```python
from build123d import *

# Parameters (mm, degrees)
CYLINDER028_R           = 1.1
CYLINDER028_DEPTH       = 10
CYLINDER031_R           = 0.9
CYLINDER031_DEPTH       = 10
CYLINDER029_R           = 2.5
CYLINDER029_DEPTH       = 3.5
CYLINDER030_R           = 2
CYLINDER030_DEPTH       = 5.2
LINK011_PLACEMENT_ANGLE = 90
LINK012_PLACEMENT_ANGLE = 90
CYLINDER027_R           = 1.1
CYLINDER027_DEPTH       = 10
CYLINDER025_R           = 1.1
CYLINDER025_DEPTH       = 10
CYLINDER026_R           = 1.1
CYLINDER026_DEPTH       = 10
LINK010_PLACEMENT_ANGLE = 90
LINK009_PLACEMENT_ANGLE = 90
CYLINDER018_R           = 3.25
CYLINDER018_DEPTH       = 10
BOX010_W                = 3.25
BOX010_H                = 9
BOX010_DEPTH            = 22
BOX009_W                = 3.25
BOX009_H                = 9
BOX009_DEPTH            = 2
CYLINDER024_R           = 5
CYLINDER024_DEPTH       = 1.5
CYLINDER023_R           = 5
CYLINDER023_DEPTH       = 1.5
CYLINDER019_R           = 3.25
CYLINDER019_DEPTH       = 10
CYLINDER004_R           = 2
CYLINDER004_DEPTH       = 40
BOX004_W                = 3.25
BOX004_H                = 24
BOX004_DEPTH            = 40


with BuildPart() as cylinder028:
    # Cylinder028 → Cylinder028 (new body)
    with BuildSketch(Plane(origin=(-3.5, 5.75, 44.25), x_dir=(0, 0, -1), z_dir=(1, 0, 0))):
        Circle(CYLINDER028_R)
    extrude(amount=CYLINDER028_DEPTH)


with BuildPart() as cylinder031:
    # Cylinder031 → Cylinder031 (new body)
    with BuildSketch(Plane.XY):
        Circle(CYLINDER031_R)
    extrude(amount=CYLINDER031_DEPTH)


with BuildPart() as cylinder029:
    # Cylinder029 → Cylinder029 (new body)
    with BuildSketch(Plane.XY):
        Circle(CYLINDER029_R)
    extrude(amount=CYLINDER029_DEPTH)


with BuildPart() as obj1:
    # Cylinder030 → Cylinder030 (new body)
    with BuildSketch(Plane.XY):
        Circle(CYLINDER030_R)
    extrude(amount=CYLINDER030_DEPTH)

    # Fusion018: union Cylinder029
    add(cylinder029.part)

    # Cut007: cut Cylinder031
    add(cylinder031.part, mode=Mode.SUBTRACT)


with BuildPart() as obj2:
    # Link011 base: copy of obj1
    add(obj1.part)


with BuildPart() as obj2_1:
    # Link011 placement: moved
    add(obj2.part.moved(Location((-2.5, -5.75, 44.25))).rotate(Axis((-2.5, -5.75, 44.25), (0, 1, 0)), LINK011_PLACEMENT_ANGLE))


with BuildPart() as obj3:
    # Link012 base: copy of obj1
    add(obj1.part)


with BuildPart() as obj3_1:
    # Link012 placement: moved
    add(obj3.part.moved(Location((-2.5, 5.75, 44.25))).rotate(Axis((-2.5, 5.75, 44.25), (0, 1, 0)), LINK012_PLACEMENT_ANGLE))


with BuildPart() as fusion017:
    # Cylinder027 → Cylinder027 (new body)
    with BuildSketch(Plane(origin=(-3.5, -5.75, 44.25), x_dir=(0, 0, -1), z_dir=(1, 0, 0))):
        Circle(CYLINDER027_R)
    extrude(amount=CYLINDER027_DEPTH)

    # Fusion017: union Cylinder028, obj2, obj3
    add(cylinder028.part)
    add(obj2_1.part)
    add(obj3_1.part)


with BuildPart() as cylinder025:
    # Cylinder025 → Cylinder025 (new body)
    with BuildSketch(Plane(origin=(-3.5, -5.75, 9.75), x_dir=(0, 0, -1), z_dir=(1, 0, 0))):
        Circle(CYLINDER025_R)
    extrude(amount=CYLINDER025_DEPTH)


with BuildPart() as cylinder026:
    # Cylinder026 → Cylinder026 (new body)
    with BuildSketch(Plane(origin=(-3.5, 5.75, 9.75), x_dir=(0, 0, -1), z_dir=(1, 0, 0))):
        Circle(CYLINDER026_R)
    extrude(amount=CYLINDER026_DEPTH)


with BuildPart() as obj4:
    # Link010 base: copy of obj1
    add(obj1.part)


with BuildPart() as obj4_1:
    # Link010 placement: moved
    add(obj4.part.moved(Location((-2.5, 5.75, 9.75))).rotate(Axis((-2.5, 5.75, 9.75), (0, 1, 0)), LINK010_PLACEMENT_ANGLE))


with BuildPart() as fusion019:
    # Link009 base: copy of obj1
    add(obj1.part)


with BuildPart() as fusion019_1:
    # Link009 placement: moved
    add(fusion019.part.moved(Location((-2.5, -5.75, 9.75))).rotate(Axis((-2.5, -5.75, 9.75), (0, 1, 0)), LINK009_PLACEMENT_ANGLE))

    # Fusion016: union Cylinder025, Cylinder026, obj4
    add(cylinder025.part)
    add(cylinder026.part)
    add(obj4_1.part)

    # Fusion019: union Fusion017
    add(fusion017.part)


with BuildPart() as cylinder018:
    # Cylinder018 → Cylinder018 (new body)
    with BuildSketch(Plane(origin=(-3.5, 7.5, 34.5), x_dir=(0, 0, -1), z_dir=(1, 0, 0))):
        Circle(CYLINDER018_R)
    extrude(amount=CYLINDER018_DEPTH)


with BuildPart() as cube010:
    # Box010 → Box010 (new body)
    with BuildSketch(Plane(origin=(-3.5, -12, 16), x_dir=(1, 0, 0), z_dir=(0, 0, 1))):
        with Locations((1.625, 4.5)):
            Rectangle(BOX010_W, BOX010_H)
    extrude(amount=BOX010_DEPTH)


with BuildPart() as cube009:
    # Box009 → Box009 (new body)
    with BuildSketch(Plane(origin=(-3.5, 3, 26), x_dir=(1, 0, 0), z_dir=(0, 0, 1))):
        with Locations((1.625, 4.5)):
            Rectangle(BOX009_W, BOX009_H)
    extrude(amount=BOX009_DEPTH)


with BuildPart() as cylinder024:
    # Cylinder024 → Cylinder024 (new body)
    with BuildSketch(Plane(origin=(-1.75, 7.5, 19.5), x_dir=(0, 0, -1), z_dir=(1, 0, 0))):
        Circle(CYLINDER024_R)
    extrude(amount=CYLINDER024_DEPTH)


with BuildPart() as fusion015:
    # Cylinder023 → Cylinder023 (new body)
    with BuildSketch(Plane(origin=(-1.75, 7.5, 34.5), x_dir=(0, 0, -1), z_dir=(1, 0, 0))):
        Circle(CYLINDER023_R)
    extrude(amount=CYLINDER023_DEPTH)

    # Fusion015: union Cylinder024
    add(cylinder024.part)


with BuildPart() as fusion011:
    # Cylinder019 → Cylinder019 (new body)
    with BuildSketch(Plane(origin=(-3.5, 7.5, 19.5), x_dir=(0, 0, -1), z_dir=(1, 0, 0))):
        Circle(CYLINDER019_R)
    extrude(amount=CYLINDER019_DEPTH)

    # Fusion011: union Cylinder018, Cube010, Cube009, Fusion015
    add(cylinder018.part)
    add(cube010.part)
    add(cube009.part)
    add(fusion015.part)


with BuildPart() as beamhole:
    # Cylinder004 → Cylinder004 (new body)
    with BuildSketch(Plane.XY):
        Circle(CYLINDER004_R)
    extrude(amount=CYLINDER004_DEPTH)


with BuildPart() as obj5:
    # Box004 → Box004 (new body)
    with BuildSketch(Plane(origin=(-3.5, -12, 0), x_dir=(1, 0, 0), z_dir=(0, 0, 1))):
        with Locations((1.625, 12)):
            Rectangle(BOX004_W, BOX004_H)
    extrude(amount=BOX004_DEPTH)

    # Cut001: cut Beamhole
    add(beamhole.part, mode=Mode.SUBTRACT)


with BuildPart() as obj5_1:
    # Cut001 placement: moved
    add(obj5.part.moved(Location((0, 0, 7))))

    # Cut005: cut Fusion011
    add(fusion011.part, mode=Mode.SUBTRACT)

    # Cut008: cut Fusion019
    add(fusion019_1.part, mode=Mode.SUBTRACT)


with BuildPart() as obj5_2:
    # Cut008 placement: moved
    add(obj5_1.part.moved(Location((0, 0, 1))))


solid = obj5_2.part
```
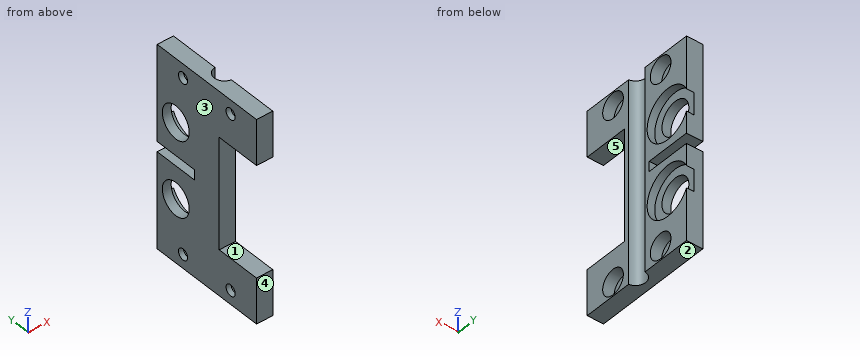
CAD build for the part. Positions are in the model's coordinates, mm. Face numbers are marked on the shaded views. A direction names the side the tool comes from. Give positions to 0.01 mm unless a question says otherwise; leave off trailing zeros. Order: outer loops, then holes, each group sorted by start corner. A loop starts at its lowest first (then second) coordinate and runs counter-clockwise, first axis right, second up. Notation, with made-up numbers: M -2,-18 L 29,-18 A18 cw 29,1 Z; hole C 78,65 d5. An arc over 180 degrees is marked long. Put each result on its own line as item: value. Start each with the question number.
(1) Saw through at A-A, the plane z = 45.25. Write the cut outline in (x, y).
(2) Drill centre lines: line 1 along Y through (x, z) = (-3.25, 10.75); line 2 along Z through (x, y) = (-2.9, -5.75); line 3 along Y through (x, z) = (-0.75, 10.75). Where is each one in solid material? Low to high.
(3) Saw through at D-D, the plane z = 35.5. Write the cut outline in (x, y), then the cut area to 3 significant figures.
(4) Which spindle directions (+Z, -Z, +X, -X, +Y, -Y) get a long thin tool onto all of the face, cutting with end or side? Do the marked faces 4 and 5. Say none if no direction does.
(5) Mould opens along Z. For the marked faces 1, 2 and 3 say: +Z half, -Z half, draft (parallel to the pull), parting line (faces both ways), or undercut.
(6) Saw through at C-C, the plane y = -5.75. Write the cut outline in (x, z), then the cut area to 3 significant figures.
(7) Flat gauge pins, fed straight in: pin 1 Ø1.5 at (y, z) = (7, 46) entering from +X; pin 2 Ø6 at (y, z) = (7.5, 20.5) entering from -X; pin 3 Ø1 at (x, z) = (-2.5, 28) entering from +Y. Where does each tip first touch, or does it go through?
(8) Saw through at B-B, the plane x = -2.9. Write the cut outline in (y, z).
Check result:
1. outline: M -3.5,-12 L -0.25,-12 L -0.25,-8.25 L -2.5,-8.25 L -2.5,-6.85 L -3.5,-6.85 Z; M -3.5,-4.65 L -2.5,-4.65 L -2.5,-3.25 L -0.25,-3.25 L -0.25,-1.98 A2 cw -0.25,1.98 L -0.25,3.25 L -2.5,3.25 L -2.5,4.65 L -3.5,4.65 Z; M -3.5,6.85 L -2.5,6.85 L -2.5,8.25 L -0.25,8.25 L -0.25,12 L -3.5,12 Z
2. line 1: y = -12 to -6.85, -4.65 to 4.65, 6.85 to 12
2. line 2: z = 8 to 9.65, 11.85 to 17, 39 to 44.15, 46.35 to 48
2. line 3: y = -12 to -8.25, -3.25 to -1.85, 1.85 to 3.25, 8.25 to 12
3. outline: M -3.5,-3 L -0.25,-3 L -0.25,-1.98 A2 cw -0.25,1.98 L -0.25,2.5 L -1.75,2.5 L -1.75,4.25 L -3.5,4.25 Z; M -3.5,10.75 L -1.75,10.75 L -1.75,12 L -3.5,12 Z
3. area: 17.8 mm2
4. face 4: +Z, -Z, +X, -X, -Y
4. face 5: +X, -X, -Y
5. face 1: undercut
5. face 2: -Z half
5. face 3: draft
6. outline: M -3.5,8 L -0.25,8 L -0.25,8.25 L -2.5,8.25 L -2.5,9.65 L -3.5,9.65 Z; M -3.5,11.85 L -2.5,11.85 L -2.5,13.25 L -0.25,13.25 L -0.25,17 L -3.5,17 Z; M -3.5,39 L -0.25,39 L -0.25,42.75 L -2.5,42.75 L -2.5,44.15 L -3.5,44.15 Z; M -3.5,46.35 L -2.5,46.35 L -2.5,47.75 L -0.25,47.75 L -0.25,48 L -3.5,48 Z
6. area: 31.6 mm2
7. pin 1: stops at x = -2.5
7. pin 2: passes through
7. pin 3: stops at y = 3
8. outline: M -12,8 L 12,8 L 12,27 L 3,27 L 3,29 L 12,29 L 12,48 L -12,48 L -12,39 L -3,39 L -3,17 L -12,17 Z; hole C -5.75,10.75 d2.2; hole C -5.75,45.25 d2.2; hole C 7.5,20.5 d6.5; hole C 7.5,35.5 d6.5; hole C 5.75,10.75 d2.2; hole C 5.75,45.25 d2.2
